Autodesk Inventor part; units mm, degrees
ref_plane "YZ Plane" through (0, 0, 0) normal (1, 0, 0) x (0, 1, 0)
ref_plane "XZ Plane" through (0, 0, 0) normal (0, 1, 0) x (-1, 0, 0)
ref_plane "XY Plane" through (0, 0, 0) normal (0, 0, 1) x (1, 0, 0)
sketch "Sketch1" plane through (0, 0, 0) normal (1, 0, 0) x (0, 1, 0)
  circle A0 centre (0, 0) radius 4
  dimension "d0" = 8
extrude "Extrusion1" add sketch "Sketch1" along normal blind 35
sketch "Sketch2" plane through (0, 0, 0) normal (-1, 0, 0) x (0, 0, 1)
  circle A0 centre (0, 0) radius 3.75
  dimension "d3" = 7.5
extrude "Extrusion2" cut sketch "Sketch2" against normal blind 0.2
sketch "Sketch3" plane through (35, 0, 0) normal (1, 0, 0) x (0, 0, -1)
  circle A0 centre (0, 0) radius 3.75
  dimension "d6" = 7.5
extrude "Extrusion3" add sketch "Sketch3" along normal blind 0.2
sketch "Sketch4" plane through (35.2, 0, 0) normal (1, 0, 0) x (0, 0, -1)
  circle A0 centre (0, 0) radius 4
  circle A1 centre (0, 0) radius 4
  dimension "d9" = 8
extrude "Extrusion4" add sketch "Sketch4" along normal blind 8
sketch "Sketch5" plane through (43.2, 0, 0) normal (1, 0, 0) x (0, 0, -1)
  circle A0 centre (0, 0) radius 2
  dimension "d12" = 4
extrude "Extrusion5" add sketch "Sketch5" along normal blind 50
properties part number "webcam_new" material "Steel, Paint Finish, Dark Gray, Matte"
Build history of the part. All positions in model axes, mm. A direction names the side the tool comes from. Round coordinates to 2 decimals unless told otherwise and drop trailing zeros. Write each loop counter-clockwise with the first axis right and the second up, starting at its lowest first coordinate (ties: lowest second). Pieces come first, ordered by that corner, then holes. Notation, with made-up numbers: (86.5, 74.5) -> (142.5, 74.5) arc R10 ccw to (142.5, 82.5) -> close; hole circle Ø4 at (87, 2.5). An arc over 180 degrees is marked (long way). Use one line per item in the form item = value.
Q1. Drill centre lines: L1, parallel to X at y = 1.5, z = -2; L2, parallel to X at y = -0.75, z = 0.25; L3, parallel to Y at x = 4.5, z = -1.25. Where is each one in solid material? Low to high.
Conclusion:
L1 = 0.2 to 43.2
L2 = 0.2 to 93.2
L3 = -3.8 to 3.8
Q2. Tool access for faces 1 (the cylindrical face through (39.144, 3.905, 0.867)), 2 (the flat face through (0.2, 0, 0)), 3 (the cylindrical face through (68, 2, 0)): list every direction of +Z, -Z, +X, -X, +Y, -Y with a clear straight run to the whole face (end or side of a thin tool).
Conclusion:
face_1 = +X, -X
face_2 = -X
face_3 = +X
Q3. Band-saw the part on C-C, the plane x = 18. Write the cut outline in (y, z), then the cut area to 3 significant figures.
Conclusion:
outline = circle Ø8 at (0, 0)
area = 50.3 mm²
Q4. Band-saw the part on A-A, the plane y = 0. Write the cut outline in (x, z).
Conclusion:
outline = (0, -4) -> (35, -4) -> (35, -3.75) -> (35.2, -3.75) -> (35.2, -4) -> (43.2, -4) -> (43.2, -2) -> (93.2, -2) -> (93.2, 2) -> (43.2, 2) -> (43.2, 4) -> (35.2, 4) -> (35.2, 3.75) -> (35, 3.75) -> (35, 4) -> (0, 4) -> (0, 3.75) -> (0.2, 3.75) -> (0.2, -3.75) -> (0, -3.75) -> close
Q5. Band-saw the part on D-D, the plane x = 69. Write the cut outline in (y, z), then the cut area to 3 significant figures.
Conclusion:
outline = circle Ø4 at (0, 0)
area = 12.6 mm²
Q6. Drop flat-ended pins along their axis: P1, Ø1, axis at y = -3, z = 3, coming from the +X side; P2, Ø1, axis at x = 49, z = -1.5, coming from the -Y side; P3, Ø3, axis at x = 44, y = -1.5, coming from the +Z side. Give the stop position or say it passes through.
Conclusion:
P1 = 43.2
P2 = -1.73
P3 = 3.99
